Part print with two shaded views. Sizes in mm from the minimum x, y, z corner. A direction names the side the tool comes from. Round coordinates to 2 decimals unless told otherwise and drop trailing zeros. Order: outer loops, then holes, each group sorted by start corner. A loop starts at its lowest first (then second) coordinate and runs counter-clockwise, first axis right, second up. Notation, with made-up numbers: M 50,60.5 L 104,60.5 A23 cw 104,76.5 Z; hole C 69,-21 d2. An arc over 180 degrees is marked long. One line per question, with ' | ' between items. Start each with the question number.
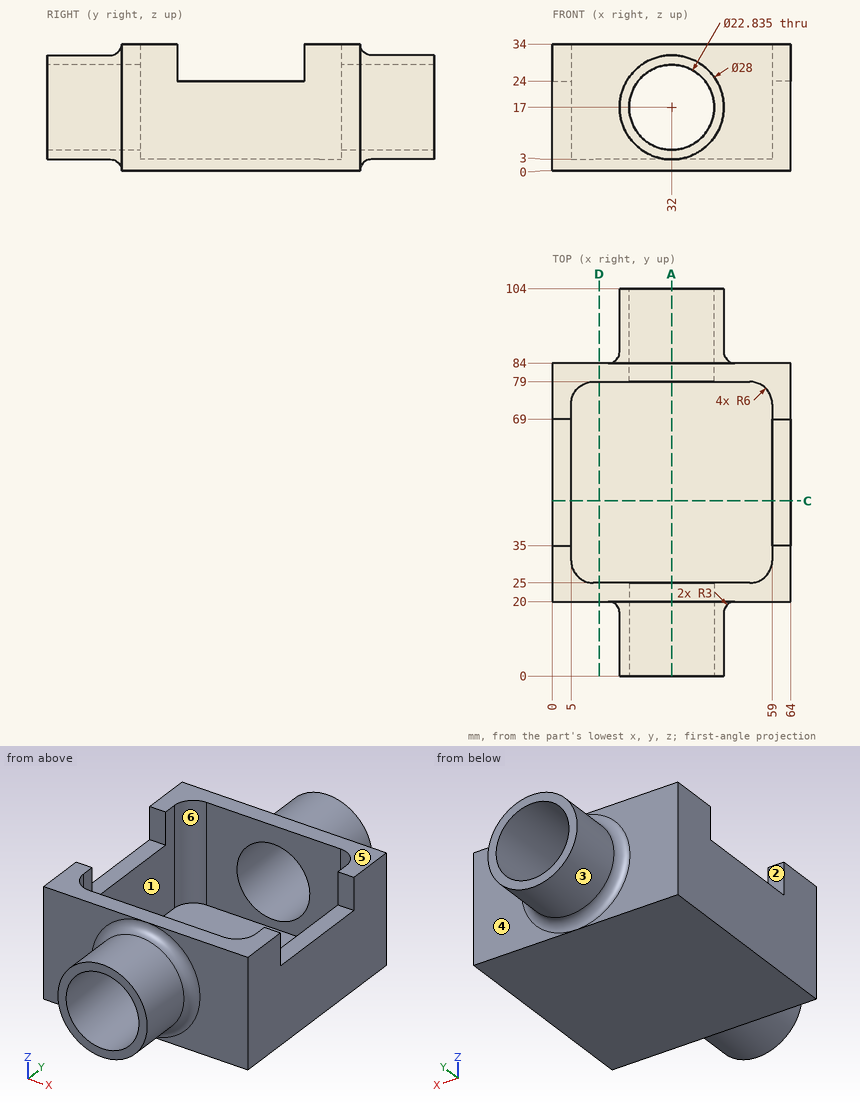
Item 1: Cut at A-A on x = 32. Count the separate pieces of the cut face and the enclosed holes in it, then the cut area to 3 significant figures.
Item 2: Wall check: line 1 along Y through (x, z) = (42.5, 24); line 2 along Y through (x, z) = (49, 18); line 3 along Z through (x, y) = (32, 16.25). Give the ranges that are in metal, low to high. Write a range as [from, to].
Item 3: Cut at C-C on y = 47. Write the cut outline in (x, z), then the cut area to 3 significant figures.
Item 4: Cut at D-D on x = 12.5. Write the cut outline in (y, z).
Item 5: Two-plate mould, pull along Y, no slides. Class the marked faces 4, 5 and 6: +Y half, -Y half, draft (parallel to the pull), parting line (faces both ways), or undercut.
Item 6: Tool access for the marked faces 1, 2 and 3: list every direction of +Z, -Z, +X, -X, +Y, -Y with a clear straight run to the whole face (end or side of a thin tool).
Item 7: Flat gauge pins, fed straight in: pin 1 (2.5 mm diameter, centred on x = 61, y = 53.5, fed in from +Z); pin 2 (1.5 mm diameter, centred on x = 62.5, z = 28, fed in from +Y); pin 3 (5.5 mm diameter, centred on x = 1.5, z = 31, fed in from -Y). Where does each tip first touch, or does it go through?
Results found:
1) separate pieces: 3 | enclosed holes: 0 | area: 488 mm^2
2) line 1: y = [0, 25], [79, 104] | line 2: y = [20, 25], [79, 84] | line 3: z = [3, 5.58], [28.42, 31]
3) outline: M 0,0 L 64,0 L 64,24 L 59,24 L 59,3 L 5,3 L 5,24 L 0,24 Z | area: 402 mm^2
4) outline: M 20,0 L 84,0 L 84,34 L 79,34 L 79,3 L 25,3 L 25,34 L 20,34 Z
5) face 4: +Y half | face 5: draft | face 6: undercut
6) face 1: +Z | face 2: +Z, +X, -X | face 3: +Y
7) pin 1: stops at z = 24 | pin 2: stops at y = 84 | pin 3: stops at y = 20
